from build123d import *

# Parameters (mm, degrees)
F1_DEPTH = 25.4
F2_R     = 6.35
F4_D     = 6
F5_R     = 6.35
F6_DEPTH = 3.171


with BuildPart() as f1:
    # F0 (on Right) → F1 (new body, symmetric)
    with BuildSketch(Plane.YZ):
        Polygon((0, 3.17), (0, 0), (25.4, 0), (25.4, 50.8), (22.23, 50.8), (22.23, 3.17), align=None)
    extrude(amount=F1_DEPTH, both=True)

    # F2
    f2_edges = [f1.edges().sort_by_distance(p)[0] for p in [
        (0, 22.23, 3.17),
    ]]
    fillet(f2_edges, radius=F2_R)

    # F4 (through all)
    with Locations(Plane.XY.offset(3.17)):
        with Locations((-12.7, 12.7), (12.7, 12.7)):
            Hole(F4_D / 2)

    # F5 (on face) → F6 (cut, through all)
    with BuildSketch(Plane.XZ.offset(-22.23)):
        with BuildLine():
            Line((-25.4, 9.52), (-11.756103, 42.904585))
            ThreePointArc((-11.756103, 42.904585), (-7.08067, 48.642965), (0, 50.8))
            Line((0, 50.8), (-25.4, 50.8))
            Line((-25.4, 50.8), (-25.4, 9.52))
        make_face()
        with BuildLine():
            ThreePointArc((0, 50.8), (7.08067, 48.642965), (11.756103, 42.904585))
            Line((11.756103, 42.904585), (25.4, 9.52))
            Line((25.4, 9.52), (25.4, 50.8))
            Line((25.4, 50.8), (0, 50.8))
        make_face()
        with Locations((0, 38.1)):
            Circle(F5_R)
    extrude(amount=-F6_DEPTH, mode=Mode.SUBTRACT)


solid = f1.part
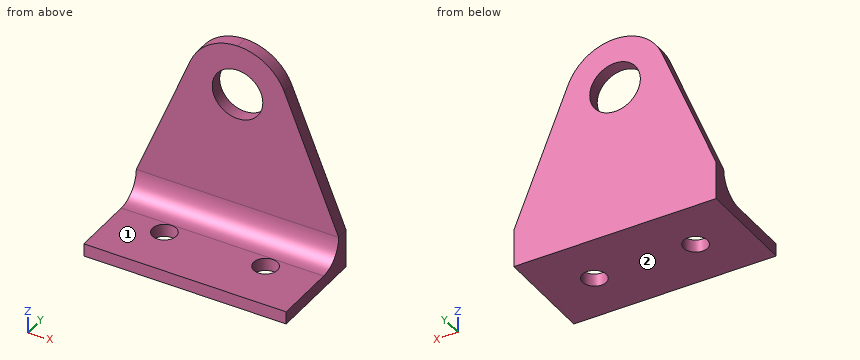
Geometry check sheet. Reference: the model listing, model coordinates, mm. Face numbers are marked on the shaded views. A direction names the side the tool comes from. Round coordinates to 2 decimals unless told otherwise and drop trailing zeros. Write each loop counter-clockwise with the first axis right and the second up, starting at its lowest first coordinate (ties: lowest second). Pieces come first, ordered by that corner, then holes.
Item 1: Section check C-C (x = 3). Record the boundary of the cut face in (y, z).
Determined:
outline: (0, 0) - (25.4, 0) - (25.4, 32.5) - (22.23, 32.5) - (22.23, 9.52) arc R6.35 cw to (15.88, 3.17) - (0, 3.17) - close; (22.23, 43.7) - (25.4, 43.7) - (25.4, 50.44) - (22.23, 50.44) - close
Item 2: Go/stop test with flat-tipped pins: pin 1 Ø5 at (x, y) = (-9, 5) entering from +Z; pin 2 Ø12 at (x, y) = (8, 12) entering from +Z; pin 3 Ø8 at (x, z) = (5.5, 34.5) entering from -Y; pin 4 Ø5.5 at (x, y) = (12.7, 12.7) entering from -Z. Record where each tip stops, or that it passes through.
Determined:
pin 1: stops at z = 3.17
pin 2: stops at z = 3.53
pin 3: stops at y = 22.23
pin 4: passes through
Item 3: Material ranges on line 1 along Z through (x, y) = (0, 24.6); line 2 along Y through (x, z) = (12.7, 1.6); line 3 along Z through (x, y) = (0, 8), recorded low to high.
Determined:
line 1: z = 0 to 31.75, 44.45 to 50.8
line 2: y = 0 to 9.7, 15.7 to 25.4
line 3: z = 0 to 3.17
Item 4: Section check D-D (x = 17). Record the boundary of the cut face in (y, z).
Determined:
outline: (0, 0) - (25.4, 0) - (25.4, 30.07) - (22.23, 30.07) - (22.23, 9.52) arc R6.35 cw to (15.88, 3.17) - (0, 3.17) - close
Item 5: Access from +Z, -Z, +X, -X, +Y, -Y to the whole of each face (thin tool, end or side, straight path). Record for the marked faces 1 and 2.
Determined:
face 1: +Z, +X, -X, -Y
face 2: -Z, +X, -X, +Y, -Y
Item 6: Section check B-B (z = 38.1). Record the boundary of the cut face in (x, y), plus the area to 3 significant figures.
Determined:
outline: (-13.72, 22.23) - (-6.35, 22.23) - (-6.35, 25.4) - (-13.72, 25.4) - close; (6.35, 22.23) - (13.72, 22.23) - (13.72, 25.4) - (6.35, 25.4) - close
area: 46.7 mm2
Item 7: Section check A-A (y = 12.7). Record the boundary of the cut face in (x, z).
Determined:
outline: (-25.4, 0) - (-15.7, 0) - (-15.7, 3.17) - (-25.4, 3.17) - close; (-9.7, 0) - (9.7, 0) - (9.7, 3.17) - (-9.7, 3.17) - close; (15.7, 0) - (25.4, 0) - (25.4, 3.17) - (15.7, 3.17) - close
